CAD build for the part. Positions are in the model's coordinates, mm. Face numbers are marked on the shaded views. Coordinates: 2 decimals unless noted, no trailing zeros. Write each loop counter-clockwise with the first axis right and the second up, starting at its lowest first coordinate (ties: lowest second). Pieces come first, ordered by that corner, then holes. Notation, with made-up numbers: (-3, -7.5) -> (4, -7.5) arc R19 ccw to (4, 15.5) -> close; hole circle Ø10 at (60.25, 2.5). An arc over 180 degrees is marked (long way). Answer as CSV lines item,"result".
```python
from build123d import *

# Parameters (mm, degrees)
SKETCH1_W                = 82
SKETCH1_H                = 683.5
BASE_FLANGE1_DEPTH       = 5
SKETCHED_START           = -41
SKETCHED_BEND1_DEPTH     = 82
SKETCHED_BEND1_2_DEPTH   = 82
M6_CLEARANCE_HOLE1_D     = 6.4
M6_CLEARANCE_HOLE1_DEPTH = 5
M6_CLEARANCE_HOLE1_TIP   = 1.922753981
SKETCH8_R                = 10.5
CUT_EXTRUDE1_DEPTH       = 373.579466057
SKETCH9_R                = 1.55
SKETCH9_W                = 71
SKETCH9_H                = 24
SKETCH9_W_2              = 10
SKETCH9_H_2              = 10
CUT_EXTRUDE2_DEPTH       = 373.579466057
M6_CLEARANCE_HOLE3_D     = 6.4
M6_CLEARANCE_HOLE3_DEPTH = 5
M6_CLEARANCE_HOLE3_TIP   = 1.922753981
M6_CLEARANCE_HOLE4_D     = 6.4
M6_CLEARANCE_HOLE4_DEPTH = 5
M6_CLEARANCE_HOLE4_TIP   = 1.922753981


# Read off the part's stored shape, not the designer's step: Sketched Bend1
# Sheet-metal steps are written as plain solids
with BuildPart() as part:
    # Sketch1 → Base-Flange1 (new body)
    with BuildSketch(Plane.XY):
        Rectangle(SKETCH1_W, SKETCH1_H)
    extrude(amount=-BASE_FLANGE1_DEPTH)

    # Sketched Bend1 outline → Sketched Bend1 (cut)
    with BuildSketch(Plane.YZ.offset(SKETCHED_START)):
        with BuildLine():
            Line((-341.75, -5), (-193.978990152, -5))
            ThreePointArc((-193.978990152, -5), (-196.17429193, -4.563327326), (-198.035378913, -3.319788761))
            Line((-198.035378913, -3.319788761), (-201.355167674, 0))
            Line((-201.355167674, 0), (-341.75, 0))
            Line((-341.75, 0), (-341.75, -5))
        make_face()
        with BuildLine():
            ThreePointArc((45.035378913, -3.319788761), (43.17429193, -4.563327326), (40.978990152, -5))
            Line((40.978990152, -5), (341.75, -5))
            Line((341.75, -5), (341.75, 0))
            Line((341.75, 0), (48.355167674, 0))
            Line((48.355167674, 0), (45.035378913, -3.319788761))
        make_face()
    extrude(amount=SKETCHED_BEND1_DEPTH, mode=Mode.SUBTRACT)

    # Sketched Bend1 2 outline → Sketched Bend1 2 (add)
    with BuildSketch(Plane.YZ.offset(SKETCHED_START)):
        with BuildLine():
            Line((-300.727782675, 99.372615001), (-201.355167674, 0))
            Line((-201.355167674, 0), (-193.978990152, 0))
            ThreePointArc((-193.978990152, 0), (-194.260874768, 0.056070336), (-194.499845007, 0.215745145))
            Line((-194.499845007, 0.215745145), (-297.192248769, 102.908148906))
            Line((-297.192248769, 102.908148906), (-300.727782675, 99.372615001))
        make_face()
        with BuildLine():
            Line((40.978990152, 0), (48.355167674, 0))
            Line((48.355167674, 0), (255.915120196, 207.559952522))
            Line((255.915120196, 207.559952522), (252.37958629, 211.095486428))
            Line((252.37958629, 211.095486428), (41.499845007, 0.215745145))
            ThreePointArc((41.499845007, 0.215745145), (41.260874768, 0.056070336), (40.978990152, 0))
        make_face()
    extrude(amount=SKETCHED_BEND1_2_DEPTH)

    # M6 Clearance Hole1
    with Locations(Plane(origin=(0, 0, -5), x_dir=(-1, 0, 0), z_dir=(0, 0, -1))):
        with Locations((-26, 26.978990152), (26, 26.978990152)):
            Hole(M6_CLEARANCE_HOLE1_D / 2, depth=M6_CLEARANCE_HOLE1_DEPTH)
            with Locations((0, 0, -(M6_CLEARANCE_HOLE1_DEPTH + M6_CLEARANCE_HOLE1_TIP / 2))):  # 118° drill point
                Cone(0, M6_CLEARANCE_HOLE1_D / 2, M6_CLEARANCE_HOLE1_TIP, mode=Mode.SUBTRACT)

    # Sketch8 → Cut-Extrude1 (cut, through all)
    with BuildSketch(Plane(origin=(0, 0, -5), x_dir=(-1, 0, 0), z_dir=(0, 0, -1))):
        with Locations((0, -9.021009848)):
            Circle(SKETCH8_R)
    extrude(amount=-CUT_EXTRUDE1_DEPTH, mode=Mode.SUBTRACT)

    # Sketch9 → Cut-Extrude2 (cut, through all)
    with BuildSketch(Plane(origin=(0, 0, -5), x_dir=(-1, 0, 0), z_dir=(0, 0, -1))):
        with Locations((-37.5, -43.521009848)):
            Circle(SKETCH9_R)
        with Locations((-37.5, -74.521009848)):
            Circle(SKETCH9_R)
        with Locations((37.5, -74.521009848)):
            Circle(SKETCH9_R)
        with Locations((37.5, -43.521009848)):
            Circle(SKETCH9_R)
        with Locations((0, -59.021009848)):
            Rectangle(SKETCH9_W, SKETCH9_H)
        with Locations((0, -86.021009848)):
            Rectangle(SKETCH9_W_2, SKETCH9_H_2)
        with Locations((-25, -86.021009848)):
            Rectangle(SKETCH9_W_2, SKETCH9_H_2)
        with Locations((25, -86.021009848)):
            Rectangle(SKETCH9_W_2, SKETCH9_H_2)
    extrude(amount=-CUT_EXTRUDE2_DEPTH, mode=Mode.SUBTRACT)

    # M6 Clearance Hole3
    with Locations(Plane(origin=(0, -100.677583837, -100.677583837), x_dir=(-1, 0, 0), z_dir=(0, -0.7071067811865487, -0.7071067811865465))):
        with Locations((-26, -207.913704352), (26, -207.913704352), (26, -267.913704352), (-26, -267.913704352)):
            Hole(M6_CLEARANCE_HOLE3_D / 2, depth=M6_CLEARANCE_HOLE3_DEPTH)
            with Locations((0, 0, -(M6_CLEARANCE_HOLE3_DEPTH + M6_CLEARANCE_HOLE3_TIP / 2))):  # 118° drill point
                Cone(0, M6_CLEARANCE_HOLE3_D / 2, M6_CLEARANCE_HOLE3_TIP, mode=Mode.SUBTRACT)

    # M6 Clearance Hole4
    with Locations(Plane(origin=(0, 24.177583837, -24.177583837), x_dir=(1, 0, 0), z_dir=(0, 0.7071067811865487, -0.7071067811865465))):
        with Locations((-26, -307.72636683), (26, -307.72636683)):
            Hole(M6_CLEARANCE_HOLE4_D / 2, depth=M6_CLEARANCE_HOLE4_DEPTH)
            with Locations((0, 0, -(M6_CLEARANCE_HOLE4_DEPTH + M6_CLEARANCE_HOLE4_TIP / 2))):  # 118° drill point
                Cone(0, M6_CLEARANCE_HOLE4_D / 2, M6_CLEARANCE_HOLE4_TIP, mode=Mode.SUBTRACT)


solid = part.part
```
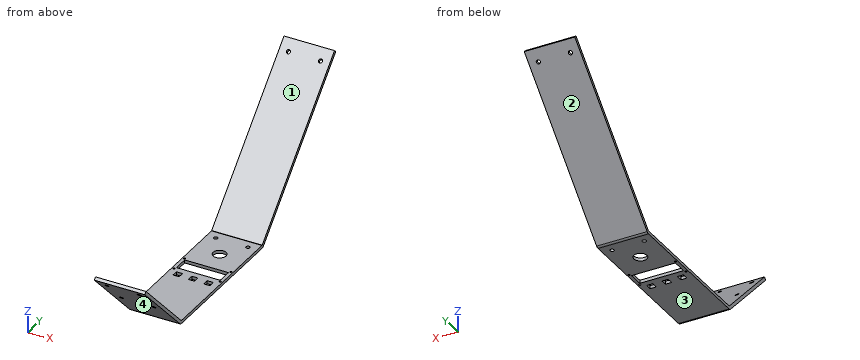
Item 1: Saw through at D-D on z = 132. Give the cut face in (x, y), and give its area (3 significant figures).
Answer below:
outline,"(-41, 173.28) -> (41, 173.28) -> (41, 180.36) -> (-41, 180.36) -> close"
area,"580 mm2"
Item 2: Two-plate mould, pull along Y, no slides. Class the marked faces 1, 2, 3 and 4: pulls with the +Y half, pulls with the -Y half, needs draft (parallel to the pull), parting line crosses it, or undercut.
Answer below:
face 1,"undercut"
face 2,"pulls with the +Y half"
face 3,"needs draft"
face 4,"pulls with the -Y half"
Item 3: Flat gauge pins, fed straight in: pin 1 (5 mm diameter, centred on x = 26, y = 26.98, fed in from +Z); pin 2 (3 mm diameter, centred on x = -7.5, y = 176, fed in from +Z); pin 3 (2.5 mm diameter, centred on x = 25.5, z = -2.5, fed in from -Y); pin 4 (12 mm diameter, centred on x = 17, z = 32.5, fed in from -Y). Where does each tip first touch, or does it go through?
Answer below:
pin 1,"passes through"
pin 2,"stops at z = 136.22"
pin 3,"stops at y = -200.11"
pin 4,"stops at y = -239.86"
Item 4: Saw through at B-B on z = 39. Give the cut face in (x, y), and give its area (3 significant figures).
Answer below:
outline,"(-41, -240.36) -> (41, -240.36) -> (41, -233.28) -> (-41, -233.28) -> close; (-41, 80.28) -> (41, 80.28) -> (41, 87.36) -> (-41, 87.36) -> close"
area,"1,160 mm2"
Item 5: Saw through at A-A on x = 0. Give the cut face in (y, z), and give its area (3 significant figures).
Answer below:
outline,"(-300.73, 99.37) -> (-198.04, -3.32) arc R5.74 ccw to (-193.98, -5) -> (-91.02, -5) -> (-91.02, 0) -> (-193.98, 0) arc R0.74 cw to (-194.5, 0.22) -> (-297.19, 102.91) -> close; (-81.02, -5) -> (-71.02, -5) -> (-71.02, 0) -> (-81.02, 0) -> close; (-47.02, -5) -> (-19.52, -5) -> (-19.52, 0) -> (-47.02, 0) -> close; (1.48, -5) -> (40.98, -5) arc R5.74 ccw to (45.04, -3.32) -> (255.92, 207.56) -> (252.38, 211.1) -> (41.5, 0.22) arc R0.74 cw to (40.98, 0) -> (1.48, 0) -> close"
area,"3,140 mm2"
Item 6: Saw through at C-C on y = 172.5. Give the cut face in (x, z), and give its area (3 significant figures).
Answer below:
outline,"(-41, 124.14) -> (41, 124.14) -> (41, 131.22) -> (-41, 131.22) -> close"
area,"580 mm2"
Item 7: Wall check: line 1 (Y direction, x = -37, z = -3); line 2 (Y direction, x = 37.5, z = -3.5); line 3 (Y direction, x = -26, z = -1.9). Give the ranges that are in metal, low to high. Write a range as from..to.
Answer below:
line 1,"y = -198.36..-75.99, -73.05..-44.99, -42.05..45.36"
line 2,"y = -197.85..-76.07, -72.97..-45.07, -41.97..44.85"
line 3,"y = -199.46..-91.02, -81.02..-71.02, -47.02..23.78, 30.18..46.46"
